from build123d import *

# Parameters (mm, degrees)
SKETCH2_R          = 1.5
CUT_EXTRUDE1_DEPTH = 10
CIRPATTERN1_COUNT  = 4
FILLET1_R          = 0.5


with BuildPart() as part:
    # Sketch1 → Revolve1 (revolve)
    with BuildSketch(Plane(origin=(0, 0, 0), x_dir=(0, 0, -1), z_dir=(1, 0, 0))):
        Polygon((1.5, 0), (1.5, 3), (3.5, 3), (3.5, 6.5), (6, 6.5), (6, 2.5), (12.3, 2.5), (12.3, 0), align=None)
    revolve(axis=Axis((0, -5.736482489, 0), (0, 1, 0)))

    # Sketch2 → Cut-Extrude1 (cut)
    with BuildSketch(Plane.XZ):
        with Locations(Location((0, -8.3, 0), (0, 0, 270))):
            Circle(SKETCH2_R)
    cut_extrude1 = extrude(amount=-CUT_EXTRUDE1_DEPTH, mode=Mode.SUBTRACT)

    # CirPattern1: Cut-Extrude1 ×4 about axis
    cirpattern1_axis = Axis((0, 0, 0), (0, 1, 0))
    for i in range(1, CIRPATTERN1_COUNT):
        add(cut_extrude1.rotate(cirpattern1_axis, i * 360 / CIRPATTERN1_COUNT), mode=Mode.SUBTRACT)

    # Fillet1
    fillet1_edges = [part.edges().sort_by_distance(p)[0] for p in [
        (0, 0, 12.3),
        (0, 2.5, 12.3),
        (0, 2.5, 6),
        (0, 6.5, 6),
        (0, 3, 3.5),
    ]]
    fillet(fillet1_edges, radius=FILLET1_R)


solid = part.part
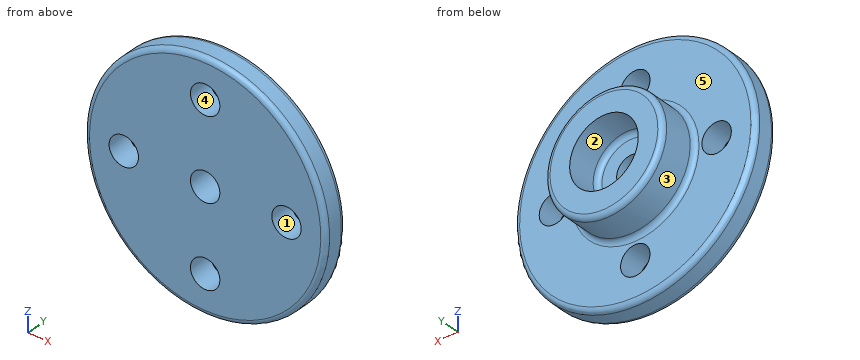
Design review of the part built by this model. Coordinates are the model's own, in mm. Face numbers are marked on the shaded views. A direction names the side the tool comes from. Round coordinates to 2 decimals unless told otherwise and drop trailing zeros. Loops run counter-clockwise (first coordinate to the right, second up) from the corner with the lowest first, then second, coordinate; pieces in that order, holes last. Notation, with made-up numbers: M 4,-31.75 L 36,-31.75 A20 cw 36,-2.75 Z; hole C 28.25,89 d7. An arc over 180 degrees is marked long. Answer as a JSON object with one key per item and string values.
Item 1: We need section A-A on z = 0. State how many separate pieces and enclosed holes the cut face has, and give its area (3 significant figures).
Answer sheet:
{"separate pieces": "4", "enclosed holes": "0", "area": "60.9 mm^2"}
Item 2: We need section C-C on y = 4.75. Give the boundary of the cut face in (x, z), and give its area (3 significant figures).
Answer sheet:
{"outline": "C 0,0 d12; hole C 0,0 d7", "area": "74.6 mm^2"}
Item 3: The part is to be moulded in two halves that separate along Z. For the marked faces 3, 4 and 5, say which applies: pulls with the +Z half, pulls with the -Z half, needs draft (parallel to the pull), parting line crosses it, or undercut.
Answer sheet:
{"face 3": "parting line crosses it", "face 4": "undercut", "face 5": "needs draft"}
Item 4: Clearance check with flat-ended pins moving along their axes: P1, Ø2.5, axis at x = -8.3, z = 0, coming from the +Y side (3 decimals); P2, Ø7, axis at x = -1.5, z = -2, coming from the +Y side; P3, Ø3, axis at x = -5.5, y = 3.5, coming from the -Z side; P4, Ø8, axis at x = -6, z = 9, coming from the +Y side. State where each tip first meets the part, or that it passes through.
Answer sheet:
{"P1": "passes through", "P2": "stops at y = 6.5", "P3": "stops at z = -11.31", "P4": "stops at y = 2.5"}
Item 5: Wall thickness on L1, parallel to X at y = 4.45, z = 0; L2, parallel to Y at x = -6.75, z = 1.25; L3, parallel to X at y = 0.75, z = 7: over which ranges is each line inside the solid? List them lowest first. Write a range as from..to.
Answer sheet:
{"L1": "x = -6..-3.5, 3.5..6", "L2": "y = 0..2.5", "L3": "x = -10.11..-0.75, 0.75..10.11"}
Item 6: Machinability: for the marked faces 1 and 2, which of the approach directions +Z, -Z, +X, -X, +Y, -Y give a long, thin tool a straight path to every point of the face, cutting with its end or side? Answer none if there is none.
Answer sheet:
{"face 1": "+Y, -Y", "face 2": "+Y"}
Item 7: We need section D-D on y = 1.5. Give the boundary of the cut face in (x, z).
Answer sheet:
{"outline": "C 0,0 d24.6; hole C -8.3,0 d3; hole C 0,-8.3 d3; hole C 0,0 d3; hole C 0,8.3 d3; hole C 8.3,0 d3"}
